Input: part model. Units: mm. Frame: model coordinates. Give positions to 0.01 mm unless a question says otherwise; leave off trailing zeros. Order: outer loops, then holes, each group sorted by start corner. A loop starts at its lowest first (then second) coordinate and runs counter-clockwise, first axis right, second up. Notation, with made-up numbers: (2, 29) - (45, 29) arc R26 ccw to (45, 61) - close; hole circle Ø4 at (11, -0.5). An arc over 180 degrees is marked (long way). Answer in a Markdown table with one row per item. Add a question column.
1. Section query B-B on y = 0.6. Return loops of the section in (x, z), and give its area (3 significant figures).
2. Section query A-A on x = 0. Return loops of the section in (y, z) (3 decimals).
3. Section query C-C on x = 5. Return loops of the section in (y, z), and give its area (3 significant figures).
4. Ray query, line 1 (Z direction, x = 0, y = 0.6); line 2 (Z direction, x = 0.75, y = 0.65); line 3 (X direction, y = 1.4, z = -0.5). Return the intervals inside material, ascending. Write a range as [from, to].
5. Section query D-D on x = -4.25. Return loops of the section in (y, z).
```python
from build123d import *

# Parameters (mm, degrees)
SKETCH1_R           = 7.94
BOSS_EXTRUDE1_DEPTH = 1.54


with BuildPart() as part:
    # Sketch1 → Boss-Extrude1 (new body)
    with BuildSketch(Plane(origin=(0, 0, 0), x_dir=(1, 0, 0), z_dir=(0, 1, 0))):
        Circle(SKETCH1_R)
        with BuildLine():
            ThreePointArc((7.94, 0), (0, -7.94), (-7.94, 0))
            Line((-7.94, 0), (-7.94, -17.5))
            Line((-7.94, -17.5), (7.94, -17.5))
            Line((7.94, -17.5), (7.94, 0))
        make_face()
    extrude(amount=BOSS_EXTRUDE1_DEPTH)

    # Sketch3 → M6 Clearance Hole1 (revolve, cut)
    with BuildSketch(Plane(origin=(0, 0, 0), x_dir=(0, 0, -1), z_dir=(1, 0, 0))):
        Polygon((0, 0), (0, 1.54), (3.3, 1.54), (3.3, 0.025), (3.325, 0), align=None)
    revolve(axis=Axis((0, -6.35, 0), (0, 1, 0)), mode=Mode.SUBTRACT)


solid = part.part
```
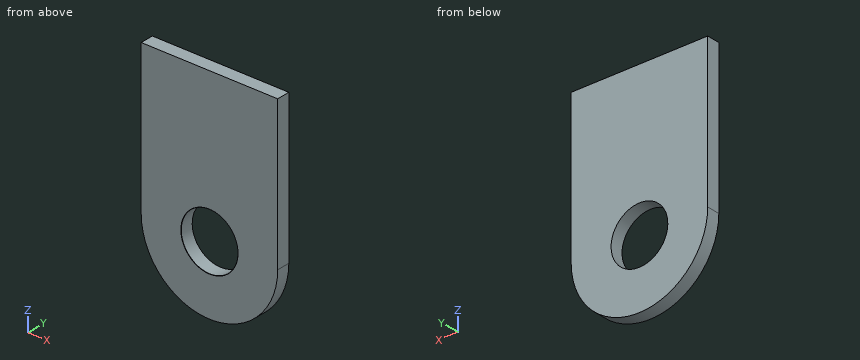
Answer:
| question | item | result |
|---|---|---|
| 1 | outline | (-7.94, 0) arc R7.94 ccw to (7.94, 0) - (7.94, 17.5) - (-7.94, 17.5) - close; hole circle Ø6.6 at (0, 0) |
| 1 | area | 343 mm² |
| 2 | outline | (0, -7.94) - (1.54, -7.94) - (1.54, -3.3) - (0.025, -3.3) - (0, -3.325) - close; (0, 3.325) - (0.025, 3.3) - (1.54, 3.3) - (1.54, 17.5) - (0, 17.5) - close |
| 3 | outline | (0, -6.17) - (1.54, -6.17) - (1.54, 17.5) - (0, 17.5) - close |
| 3 | area | 36.4 mm² |
| 4 | line 1 | z = [-7.94, -3.3], [3.3, 17.5] |
| 4 | line 2 | z = [-7.9, -3.21], [3.21, 17.5] |
| 4 | line 3 | x = [-7.92, -3.26], [3.26, 7.92] |
| 5 | outline | (0, -6.71) - (1.54, -6.71) - (1.54, 17.5) - (0, 17.5) - close |
